CAD build for the part. Positions are in the model's coordinates, mm. Coordinates: 2 decimals unless noted, no trailing zeros. Loops run counter-clockwise (first coordinate to the right, second up) from the corner with the lowest first, then second, coordinate; pieces in that order, holes last. Notation, with made-up numbers: (23, -21) - (63, -21) arc R21 cw to (63, -4) - close; hole circle Ø10 at (15.25, 45.25). An arc over 180 degrees is marked (long way). Put each result on its own line as item: value.
```python
from build123d import *

# Parameters (mm, degrees)
EXTRUDE_1_DEPTH      = 4
L298N_R              = 1.75
CUT_EXTRUDE_5_DEPTH  = 10
SKETCH_583_R         = 1.75
CUT_EXTRUDE_7_DEPTH  = 10
SKETCH_1386_W        = 40
SKETCH_1386_H        = 65
CUT_EXTRUDE_8_DEPTH  = 10
SKETCH_4195_R        = 2
CUT_EXTRUDE_10_DEPTH = 10
SKETCH_2209_R        = 1.75
SKETCH_2209_R_2      = 4.9
CUT_EXTRUDE_3_DEPTH  = 10
CUT_EXTRUDE_11_REACH = 358.759
SKETCH_11_R          = 1.75
SKETCH_12_W          = 60
SKETCH_12_H          = 40
SKETCH_12_H_2        = 10
CUT_EXTRUDE_12_DEPTH = 10
SKETCH_13_R          = 1.75
CUT_EXTRUDE_14_DEPTH = 357.758930871
SKETCH_14_R          = 1.75
CUT_EXTRUDE_15_DEPTH = 10
CUT_EXTRUDE_16_DEPTH = 10
CUT_EXTRUDE_17_DEPTH = 10


with BuildPart() as part:
    # 草图3 → 凸台-拉伸1 (new body)
    with BuildSketch(Plane.XY):
        with BuildLine():
            Line((73.505746565, 259.089488009), (196.937204075, 259.089488009))
            ThreePointArc((196.937204075, 259.089488009), (204.590872722, 257.56707866), (211.079339699, 253.231623633))
            Line((211.079339699, 253.231623633), (239.363610946, 224.947352386))
            ThreePointArc((239.363610946, 224.947352386), (243.699065973, 218.458885409), (245.221475323, 210.805216762))
            Line((245.221475323, 210.805216762), (245.221475323, 54.089488009))
            ThreePointArc((245.221475323, 54.089488009), (239.363610946, 39.947352386), (225.221475323, 34.089488009))
            Line((225.221475323, 34.089488009), (45.221475318, 34.089488009))
            ThreePointArc((45.221475318, 34.089488009), (31.079339694, 39.947352386), (25.221475318, 54.089488009))
            Line((25.221475318, 54.089488009), (25.221475318, 210.805216762))
            ThreePointArc((25.221475318, 210.805216762), (26.743884667, 218.458885409), (31.079339694, 224.947352386))
            Line((31.079339694, 224.947352386), (59.363610941, 253.231623633))
            ThreePointArc((59.363610941, 253.231623633), (65.852077918, 257.56707866), (73.505746565, 259.089488009))
        make_face()
    extrude(amount=EXTRUDE_1_DEPTH)

    # L298N → 切除-拉伸5 (cut)
    with BuildSketch(Plane.XY):
        with Locations((47.555746565, 165.855216762)):
            Circle(L298N_R)
        with Locations((47.555746565, 202.455216762)):
            Circle(L298N_R)
        with Locations((84.155746565, 202.455216762)):
            Circle(L298N_R)
        with Locations((84.155746565, 165.855216762)):
            Circle(L298N_R)
    extrude(amount=CUT_EXTRUDE_5_DEPTH, mode=Mode.SUBTRACT)

    # Sketch 583 → 切除-拉伸7 (cut)
    with BuildSketch(Plane.XY):
        with Locations((168.22147532, 227.947352386)):
            Circle(SKETCH_583_R)
        with Locations(Location((168.22147532, 151.947352386, 0), (0, 0, 180))):
            Circle(SKETCH_583_R)
        with Locations((102.22147532, 151.947352386)):
            Circle(SKETCH_583_R)
        with Locations(Location((102.22147532, 227.947352386, 0), (0, 0, 180))):
            Circle(SKETCH_583_R)
    extrude(amount=CUT_EXTRUDE_7_DEPTH, mode=Mode.SUBTRACT)

    # Sketch 1386 → 切除-拉伸8 (cut)
    with BuildSketch(Plane.XY.offset(4)):
        with Locations((225.221475323, 117.447352386)):
            Rectangle(SKETCH_1386_W, SKETCH_1386_H)
        with Locations((45.221475318, 117.447352386)):
            Rectangle(SKETCH_1386_W, SKETCH_1386_H)
    extrude(amount=-CUT_EXTRUDE_8_DEPTH, mode=Mode.SUBTRACT)

    # Sketch 4195 → 切除-拉伸10 (cut)
    with BuildSketch(Plane.XY):
        with Locations((117.72147532, 224.089488009)):
            Circle(SKETCH_4195_R)
        with Locations((152.72147532, 224.089488009)):
            Circle(SKETCH_4195_R)
    extrude(amount=CUT_EXTRUDE_10_DEPTH, mode=Mode.SUBTRACT)

    # Sketch 2209 → 切除-拉伸3 (cut)
    with BuildSketch(Plane.XY):
        with Locations(Location((185.371475323, 109.447352386, 0), (0, 0, 180))):
            Circle(SKETCH_2209_R)
        with Locations((199.371475323, 125.447352386)):
            Circle(SKETCH_2209_R)
        with Locations((192.371475323, 117.447352386)):
            Circle(SKETCH_2209_R_2)
        with Locations((185.371475323, 125.447352386)):
            Circle(SKETCH_2209_R)
        with Locations(Location((199.371475323, 109.447352386, 0), (0, 0, 180))):
            Circle(SKETCH_2209_R)
        with Locations((71.071475318, 109.447352386)):
            Circle(SKETCH_2209_R)
        with Locations(Location((85.071475318, 125.447352386, 0), (0, 0, 180))):
            Circle(SKETCH_2209_R)
        with Locations(Location((78.071475318, 117.447352386, 0), (0, 0, 180))):
            Circle(SKETCH_2209_R_2)
        with Locations(Location((71.071475318, 125.447352386, 0), (0, 0, 180))):
            Circle(SKETCH_2209_R)
        with Locations((85.071475318, 109.447352386)):
            Circle(SKETCH_2209_R)
    extrude(amount=CUT_EXTRUDE_3_DEPTH, mode=Mode.SUBTRACT)

    # 草图11 → 切除-拉伸11 (cut, up to next)
    with BuildSketch(Plane.XY.offset(4), mode=Mode.PRIVATE) as cut_extrude_11_sk1:
        with Locations((75.852077918, 90.089488009)):
            Circle(SKETCH_11_R)
    cut_extrude_11_tool1 = extrude(cut_extrude_11_sk1.sketch, amount=-CUT_EXTRUDE_11_REACH, mode=Mode.PRIVATE) & part.part
    # 草图11 → 切除-拉伸11 (cut, up to next)
    with BuildSketch(Plane.XY.offset(4), mode=Mode.PRIVATE) as cut_extrude_11_sk2:
        with Locations((70.852077918, 218.458885409)):
            Circle(SKETCH_11_R)
    cut_extrude_11_tool2 = extrude(cut_extrude_11_sk2.sketch, amount=-CUT_EXTRUDE_11_REACH, mode=Mode.PRIVATE) & part.part
    # 草图11 → 切除-拉伸11 (cut, up to next)
    with BuildSketch(Plane.XY.offset(4), mode=Mode.PRIVATE) as cut_extrude_11_sk3:
        with Locations((199.590872722, 218.458885409)):
            Circle(SKETCH_11_R)
    cut_extrude_11_tool3 = extrude(cut_extrude_11_sk3.sketch, amount=-CUT_EXTRUDE_11_REACH, mode=Mode.PRIVATE) & part.part
    # 草图11 → 切除-拉伸11 (cut, up to next)
    with BuildSketch(Plane.XY.offset(4), mode=Mode.PRIVATE) as cut_extrude_11_sk4:
        with Locations((194.590872722, 90.089488009)):
            Circle(SKETCH_11_R)
    cut_extrude_11_tool4 = extrude(cut_extrude_11_sk4.sketch, amount=-CUT_EXTRUDE_11_REACH, mode=Mode.PRIVATE) & part.part
    add(cut_extrude_11_tool1.solids().sort_by_distance((75.852078, 90.089488, 4))[0], mode=Mode.SUBTRACT)
    add(cut_extrude_11_tool2.solids().sort_by_distance((70.852078, 218.458885, 4))[0], mode=Mode.SUBTRACT)
    add(cut_extrude_11_tool3.solids().sort_by_distance((199.590873, 218.458885, 4))[0], mode=Mode.SUBTRACT)
    add(cut_extrude_11_tool4.solids().sort_by_distance((194.590873, 90.089488, 4))[0], mode=Mode.SUBTRACT)

    # 草图12 → 切除-拉伸12 (cut)
    with BuildSketch(Plane.XY.offset(4)):
        with Locations((135.22147532, 54.089488009)):
            Rectangle(SKETCH_12_W, SKETCH_12_H)
        with Locations((135.22147532, 79.089488009)):
            Rectangle(SKETCH_12_W, SKETCH_12_H_2)
    extrude(amount=-CUT_EXTRUDE_12_DEPTH, mode=Mode.SUBTRACT)

    # 草图13 → 切除-拉伸14 (cut, through all)
    with BuildSketch(Plane.XY.offset(4)):
        with Locations((83.07147532, 48.589488009)):
            Circle(SKETCH_13_R)
        with Locations((71.07147532, 48.589488009)):
            Circle(SKETCH_13_R)
        with Locations(Location((71.07147532, 79.589488009, 0), (0, 0, 180))):
            Circle(SKETCH_13_R)
        with Locations(Location((83.07147532, 79.589488009, 0), (0, 0, 180))):
            Circle(SKETCH_13_R)
        with Locations((189.22147532, 79.589488009)):
            Circle(SKETCH_13_R)
        with Locations((201.22147532, 79.589488009)):
            Circle(SKETCH_13_R)
        with Locations(Location((201.22147532, 48.589488009, 0), (0, 0, 180))):
            Circle(SKETCH_13_R)
        with Locations(Location((189.22147532, 48.589488009, 0), (0, 0, 180))):
            Circle(SKETCH_13_R)
    extrude(amount=-CUT_EXTRUDE_14_DEPTH, mode=Mode.SUBTRACT)

    # 草图14 → 切除-拉伸15 (cut)
    with BuildSketch(Plane.XY.offset(4)):
        with BuildLine():
            Line((103.22147532, 213.947352386), (101.22147532, 213.947352386))
            ThreePointArc((101.22147532, 213.947352386), (98.393048195, 212.77577951), (97.22147532, 209.947352386))
            Line((97.22147532, 209.947352386), (97.22147532, 131.947352386))
            ThreePointArc((97.22147532, 131.947352386), (98.393048195, 129.118925261), (101.22147532, 127.947352386))
            Line((101.22147532, 127.947352386), (103.22147532, 127.947352386))
            ThreePointArc((103.22147532, 127.947352386), (106.049902445, 129.118925261), (107.22147532, 131.947352386))
            Line((107.22147532, 131.947352386), (107.22147532, 209.947352386))
            ThreePointArc((107.22147532, 209.947352386), (106.049902445, 212.77577951), (103.22147532, 213.947352386))
        make_face()
        with BuildLine():
            Line((167.22147532, 213.947352386), (169.22147532, 213.947352386))
            ThreePointArc((169.22147532, 213.947352386), (172.049902445, 212.77577951), (173.22147532, 209.947352386))
            Line((173.22147532, 209.947352386), (173.22147532, 131.947352386))
            ThreePointArc((173.22147532, 131.947352386), (172.049902445, 129.118925261), (169.22147532, 127.947352386))
            Line((169.22147532, 127.947352386), (167.22147532, 127.947352386))
            ThreePointArc((167.22147532, 127.947352386), (164.393048195, 129.118925261), (163.22147532, 131.947352386))
            Line((163.22147532, 131.947352386), (163.22147532, 209.947352386))
            ThreePointArc((163.22147532, 209.947352386), (164.393048195, 212.77577951), (167.22147532, 213.947352386))
        make_face()
        with Locations((102.22147532, 207.947352386)):
            Circle(SKETCH_14_R)
    extrude(amount=-CUT_EXTRUDE_15_DEPTH, mode=Mode.SUBTRACT)

    # 草图16 → 切除-拉伸16 (cut)
    with BuildSketch(Plane.XY):
        with BuildLine():
            Line((38.186724359, 149.947352386), (38.152623691, 213.731017405))
            ThreePointArc((38.152623691, 213.731017405), (38.912804296, 217.560728224), (41.08155445, 220.807431517))
            Line((41.08155445, 220.807431517), (58.434678753, 238.160555821))
            ThreePointArc((58.434678753, 238.160555821), (61.678912242, 240.328283334), (65.505746565, 241.089488009))
            Line((65.505746565, 241.089488009), (204.937204075, 241.089488009))
            ThreePointArc((204.937204075, 241.089488009), (208.764038399, 240.328283334), (212.008271887, 238.160555821))
            Line((212.008271887, 238.160555821), (229.361396191, 220.807431517))
            ThreePointArc((229.361396191, 220.807431517), (231.530146344, 217.560728224), (232.29032695, 213.731017405))
            Line((232.29032695, 213.731017405), (232.256226281, 149.947352386))
            Line((232.256226281, 149.947352386), (245.221475323, 149.947352386))
            Line((245.221475323, 149.947352386), (245.221475323, 210.805216762))
            ThreePointArc((245.221475323, 210.805216762), (243.699065973, 218.458885409), (239.363610946, 224.947352386))
            Line((239.363610946, 224.947352386), (211.079339699, 253.231623633))
            ThreePointArc((211.079339699, 253.231623633), (204.590872722, 257.56707866), (196.937204075, 259.089488009))
            Line((196.937204075, 259.089488009), (73.505746565, 259.089488009))
            ThreePointArc((73.505746565, 259.089488009), (65.852077918, 257.56707866), (59.363610941, 253.231623633))
            Line((59.363610941, 253.231623633), (31.079339694, 224.947352386))
            ThreePointArc((31.079339694, 224.947352386), (26.743884667, 218.458885409), (25.221475318, 210.805216762))
            Line((25.221475318, 210.805216762), (25.221475318, 149.947352386))
            Line((25.221475318, 149.947352386), (38.186724359, 149.947352386))
        make_face()
    extrude(amount=CUT_EXTRUDE_16_DEPTH, mode=Mode.SUBTRACT)

    # 草图18 → 切除-拉伸17 (cut)
    with BuildSketch(Plane.XY):
        with BuildLine():
            Line((48.186724359, 44.089488009), (95.22147532, 44.089488009))
            Line((95.22147532, 44.089488009), (105.22147532, 44.089488009))
            Line((105.22147532, 44.089488009), (105.22147532, 34.089488009))
            Line((105.22147532, 34.089488009), (45.221475318, 34.089488009))
            ThreePointArc((45.221475318, 34.089488009), (31.079339694, 39.947352386), (25.221475318, 54.089488009))
            Line((25.221475318, 54.089488009), (25.221475318, 84.947352386))
            Line((25.221475318, 84.947352386), (38.186724359, 84.947352386))
            Line((38.186724359, 84.947352386), (38.186724359, 54.089488009))
            ThreePointArc((38.186724359, 54.089488009), (41.115656548, 47.018420197), (48.186724359, 44.089488009))
        make_face()
        with BuildLine():
            Line((175.22147532, 44.089488009), (222.256226281, 44.089488009))
            ThreePointArc((222.256226281, 44.089488009), (229.327294093, 47.018420197), (232.256226281, 54.089488009))
            Line((232.256226281, 54.089488009), (232.256226281, 84.947352386))
            Line((232.256226281, 84.947352386), (245.221475323, 84.947352386))
            Line((245.221475323, 84.947352386), (245.221475323, 54.089488009))
            ThreePointArc((245.221475323, 54.089488009), (239.363610946, 39.947352386), (225.221475323, 34.089488009))
            Line((225.221475323, 34.089488009), (165.22147532, 34.089488009))
            Line((165.22147532, 34.089488009), (165.22147532, 44.089488009))
            Line((165.22147532, 44.089488009), (175.22147532, 44.089488009))
        make_face()
    extrude(amount=CUT_EXTRUDE_17_DEPTH, mode=Mode.SUBTRACT)


solid = part.part
```
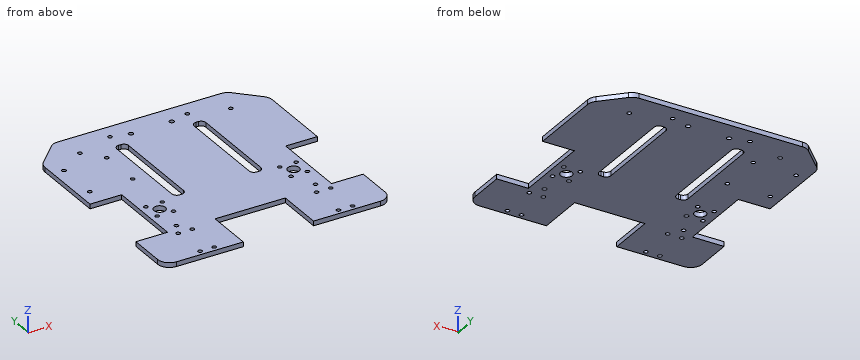
Q1. Slice it at A-A, the plane y = 175. Give the cut face in (x, z), then the cut area to 3 significant figures.
Determined:
outline: (38.17, 0) - (97.22, 0) - (97.22, 4) - (38.17, 4) - close; (107.22, 0) - (163.22, 0) - (163.22, 4) - (107.22, 4) - close; (173.22, 0) - (232.27, 0) - (232.27, 4) - (173.22, 4) - close
area: 696 mm2
Q2. Slice it at C-C, the plane x = 52.5. Give the cut face in (y, z), then the cut area to 3 significant figures.
Determined:
outline: (44.09, 0) - (84.95, 0) - (84.95, 4) - (44.09, 4) - close; (149.95, 0) - (232.23, 0) - (232.23, 4) - (149.95, 4) - close
area: 493 mm2
Q3. Pin check, flat tips, straight feed: pin 1 Ø3 at (x, y) = (83.07, 79.59) entering from +Z; pin 2 Ø2 at (x, z) = (46.5, 3) entering from -Y; pin 3 Ø2 at (y, z) = (76.5, 2) entering from -X; pin 4 Ø1.5 at (y, z) = (189.5, 3) entering from +X. Stop position of each tip, or through.
Determined:
pin 1: through
pin 2: y = 44.11
pin 3: x = 38.19
pin 4: x = 232.28
Q4. Slice it at B-B, the plane y = 63.5. Give the cut face in (x, z).
Determined:
outline: (38.19, 0) - (105.22, 0) - (105.22, 4) - (38.19, 4) - close; (165.22, 0) - (232.26, 0) - (232.26, 4) - (165.22, 4) - close
Q5. Slice it at D-D, the plane x = 158. Give the cut face in (y, z).
Determined:
outline: (84.09, 0) - (241.09, 0) - (241.09, 4) - (84.09, 4) - close
Q6. Wall check: L1, parallel to X at y = 207, z = 2.7; L2, parallel to Y at x = 76.5, z = 3.75; L3, parallel to X at y = 62.5, z = 0.6. Give the ranges that are in metal, low to high. Write a range as from..to.
Determined:
L1: 38.16..97.22, 107.22..163.22, 173.22..232.29
L2: 44.09..88.46, 91.72..112.81, 122.09..241.09
L3: 38.19..105.22, 165.22..232.26
